Job drawing, mm, ordinate dimensions from the low corner. One solid piece. A direction names the side the tool comes from. Give positions to 0.01 mm unless a question says otherwise; leave off trailing zeros. Order: outer loops, then holes, each group sorted by start corner. A loop starts at its lowest first (then second) coordinate and runs counter-clockwise, first axis right, second up. Notation, with made-up numbers: (45.25, 55.5) -> (60.25, 55.5) arc R27 ccw to (60.25, 77.5) -> close; hole circle Ø9 at (-15, 30.25). An arc over 180 degrees is marked (long way). Write item = value, one per line. Start each with the question number.
(1) Two-plate mould, pull along X, no slides. Class the marked faces 1, 2 and 3: pulls with the +X half, pulls with the -X half, needs draft (parallel to the pull), parting line crosses it, or undercut.
(2) Probe line 1 along X through (y, z) = (12, 48) (1 decimal); line 2 along Z through (x, y) = (41, 21); line 3 along Y through (x, z) = (4.5, 23). List the from-to ranges inside material, lowest first. Write a range as from..to.
(3) Saw through at C-C, the plane x = 49. List the corners of the cut face in (y, z) (1 decimal), then the cut area to 3 significant figures.
(4) Saw through at A-A, the plane z = 43.5. List the corners of the cut face in (x, y) (1 decimal), then the cut area to 3 significant figures.
(5) Saw through at B-B, the plane y = 14.5. List the corners of the cut face in (x, z) (1 decimal).
(6) Flat gauge pins, fed straight in: pin 1 (1.5 mm diameter, centred on x = 63, y = 23.5, fed in from +Z); pin 2 (3 mm diameter, centred on x = 7.5, z = 43, fed in from +Y); pin 3 (12 mm diameter, centred on y = 29, z = 24, fed in from +X); pin 4 (14.5 mm diameter, centred on x = 40, y = 6, fed in from +Z). Where does each tip first touch, or does it go through?
(7) Which spindle directions (+Z, -Z, +X, -X, +Y, -Y) get a long thin tool onto all of the face, cutting with end or side? Do the marked faces 4, 5 and 6. Say none if no direction does.
(8) Saw through at D-D, the plane z = 36. List the corners of the cut face in (x, y).
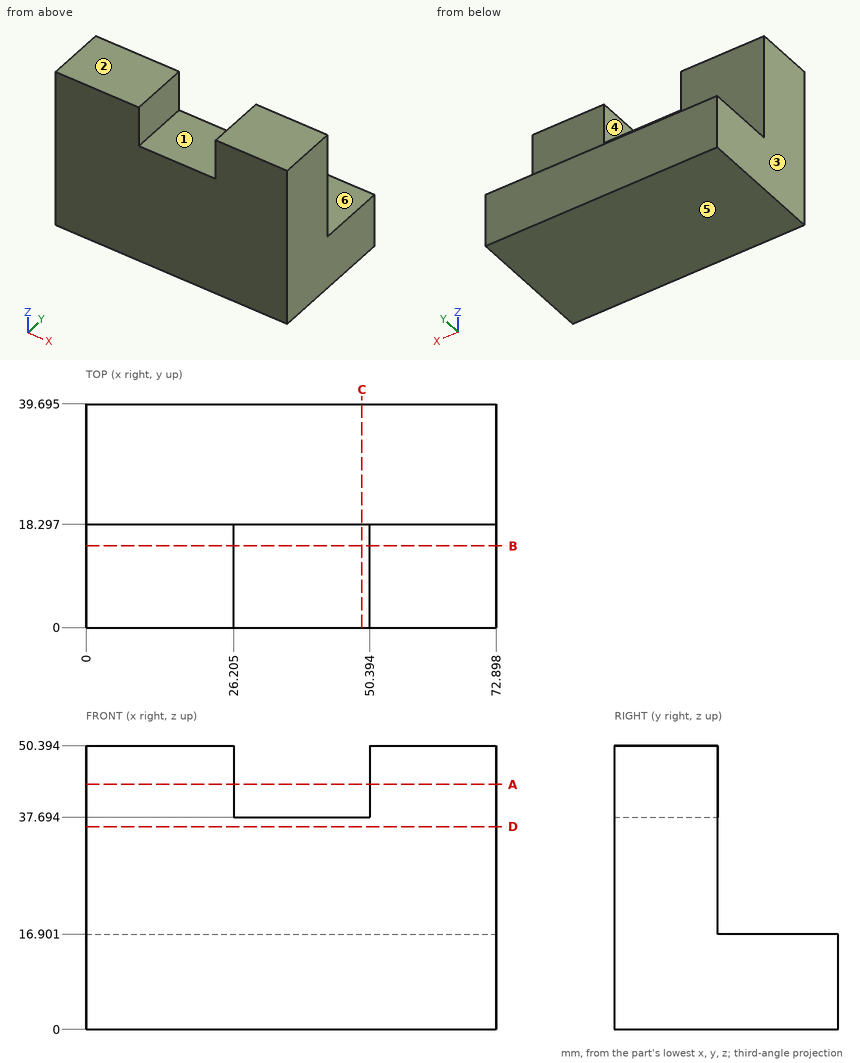
Results list:
q1.face_1 = undercut
q1.face_2 = needs draft
q1.face_3 = pulls with the -X half
q2.line_1 = 0..26.2, 50.4..72.9
q2.line_2 = 0..16.9
q2.line_3 = 0..18.3
q3.outline = (0, 0) -> (39.7, 0) -> (39.7, 16.9) -> (18.3, 16.9) -> (18.3, 37.7) -> (0, 37.7) -> close
q3.area = 1,050 mm^2
q4.outline = (0, 0) -> (26.2, 0) -> (26.2, 18.3) -> (0, 18.3) -> close; (50.4, 0) -> (72.9, 0) -> (72.9, 18.3) -> (50.4, 18.3) -> close
q4.area = 891 mm^2
q5.outline = (0, 0) -> (72.9, 0) -> (72.9, 50.4) -> (50.4, 50.4) -> (50.4, 37.7) -> (26.2, 37.7) -> (26.2, 50.4) -> (0, 50.4) -> close
q6.pin_1 = 16.9
q6.pin_2 = 18.3
q6.pin_3 = through
q6.pin_4 = 37.69
q7.face_4 = +Z, +Y, -Y
q7.face_5 = -Z, +X, -X, +Y, -Y
q7.face_6 = +Z, +X, -X, +Y
q8.outline = (0, 0) -> (72.9, 0) -> (72.9, 18.3) -> (0, 18.3) -> close
